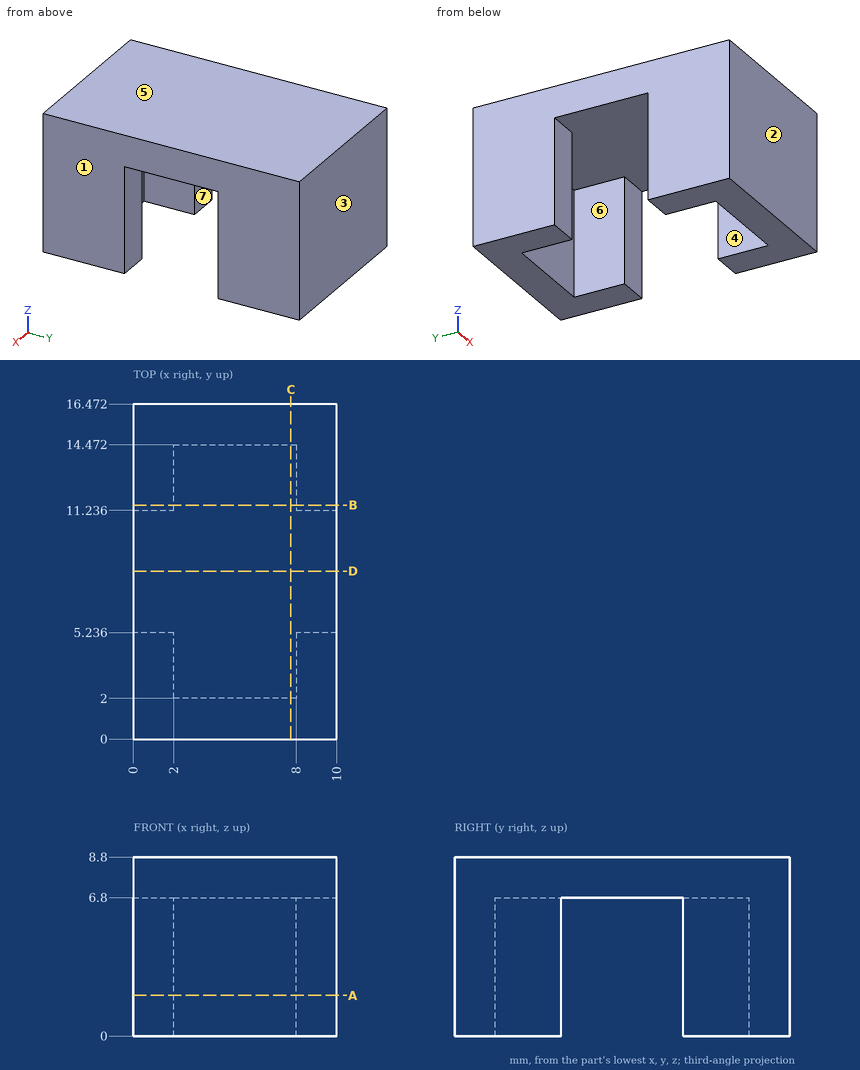
Study the drawing (mm; zero at the part's minimum x, y, z) and answer. A direction names the side the tool comes from. Give positions to 0.01 mm unless a question says otherwise; leave off trailing zeros. Order: outer loops, then holes, each group sorted by start corner. A loop starts at its lowest first (then second) coordinate and runs counter-clockwise, first axis right, second up.
1. Section C-C, the plane x = 7.75 is taken. Determine the outline of the cut face in (y, z), and give its area (3 significant figures).
Result sheet:
outline: (0, 0) - (2, 0) - (2, 6.8) - (14.47, 6.8) - (14.47, 0) - (16.47, 0) - (16.47, 8.8) - (0, 8.8) - close
area: 60.1 mm2
2. Section A-A, the plane z = 2 is taken. Determine the outline of the cut face in (x, y), and give its area (3 significant figures).
Result sheet:
outline: (0, 0) - (10, 0) - (10, 5.24) - (8, 5.24) - (8, 2) - (2, 2) - (2, 5.24) - (0, 5.24) - close; (0, 11.24) - (2, 11.24) - (2, 14.47) - (8, 14.47) - (8, 11.24) - (10, 11.24) - (10, 16.47) - (0, 16.47) - close
area: 65.9 mm2
3. Section D-D, the plane y = 8.25 is taken. Determine the outline of the cut face in (x, z), and give its area (3 significant figures).
Result sheet:
outline: (0, 6.8) - (10, 6.8) - (10, 8.8) - (0, 8.8) - close
area: 20.0 mm2
4. For the marked faces 5, 6 and 7, determine the directions among +Z, -Z, +X, -X, +Y, -Y from which every point of the face is accessible in a straight line to the end or side of a thin tool.
Result sheet:
face 5: +Z, +X, -X, +Y, -Y
face 6: -Z
face 7: -Z, +X, -X
5. This flat-tipped pin is pushed along its axis until it touches: P1, Ø1.6, axis at y = 3, z = 4.5, coming from the -X side. Where does it stop, or does it pass through?
Result sheet:
P1: stops at x = 0
6. Straight lines are drawn through the part: L1, parallel to Y at x = 5, z = 5.5; L2, parallel to X at y = 3.75, z = 4.75; L3, parallel to Y at x = 1.5, z = 6. For each, find the intervals that lie inside material, in ascending order.
Result sheet:
L1: y = 0 to 2, 14.47 to 16.47
L2: x = 0 to 2, 8 to 10
L3: y = 0 to 5.24, 11.24 to 16.47
7. Section B-B, the plane y = 11.5 is taken. Determine the outline of the cut face in (x, z), and give its area (3 significant figures).
Result sheet:
outline: (0, 0) - (2, 0) - (2, 6.8) - (8, 6.8) - (8, 0) - (10, 0) - (10, 8.8) - (0, 8.8) - close
area: 47.2 mm2
8. The mould has two halves that part along Y. Classify the marked faces 1, 2, 3 and 4: released by +Y, released by -Y, zero draft, split by the parting line, or undercut.
Result sheet:
face 1: zero draft
face 2: released by -Y
face 3: released by +Y
face 4: undercut
